For this review, take the finished solid that the model builds, in its own axes (mm). Face numbers are marked on the shaded views. A direction names the side the tool comes from. Coordinates: 2 decimals unless noted, no trailing zeros. Write each loop counter-clockwise with the first axis right and the second up, starting at its lowest first coordinate (ties: lowest second). Pieces come first, ordered by that corner, then holes.
1) We need section A-A on x = -0.5. Write out the cut boundary in (y, z).
2) We need section D-D on z = -57.5. Write out the cut boundary in (x, y), then the cut area to 3 significant figures.
3) To check wall thickness, follow line 1 along Y through (x, z) = (-0.5, 7); line 2 along Z through (x, y) = (-3.25, 13); line 3 along Y through (x, z) = (6.5, -11). State the ranges of each line that lie inside material, in increasing order.
4) For the marked faces 1, 2 and 3, list the 3-axis set-ups (+Z, -Z, +X, -X, +Y, -Y) from which the entire face can be reached by the end or side of a thin tool; tool diameter is ignored.
5) We need section B-B on z = -16. Write out the cut boundary in (x, y).
6) Insertion check: P1, Ø5, axis at x = -2.5, y = 17.5, coming from the -Z side; P2, Ø4, axis at x = 1, y = 26, coming from the -Z side; P3, Ø2, axis at x = 3.5, y = 24, coming from the +Z side. Each pin has a flat end and moves straight along its axis. Give the tip position at first contact, or say it passes through.
7) We need section C-C on y = 6. Write out the cut boundary in (x, z), then the cut area to 3 significant figures.
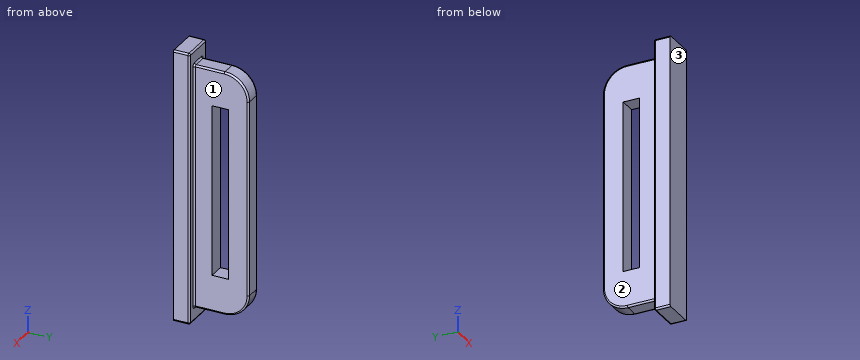
Autodesk Inventor part; units mm, degrees
ref_plane "YZ Plane" through (0, 0, 0) normal (1, 0, 0) x (0, 1, 0)
ref_plane "XZ Plane" through (0, 0, 0) normal (0, 1, 0) x (-1, 0, 0)
ref_plane "XY Plane" through (0, 0, 0) normal (0, 0, 1) x (1, 0, 0)
sketch "Sketch1" plane through (0, 0, 0) normal (1, 0, 0) x (0, 1, 0)
  line L0 (0, 76.2) -> (19.05, 76.2)
  line L1 (34.29, 60.96) -> (34.29, -60.96)
  line L2 (19.05, -76.2) -> (0, -76.2)
  line L3 (0, -76.2) -> (0, 76.2)
  line L4 (21.59, 53.34) -> (11.43, 53.34)
  line L5 (11.43, 53.34) -> (11.43, -53.34)
  line L6 (11.43, -53.34) -> (21.59, -53.34)
  line L7 (21.59, -53.34) -> (21.59, 53.34)
  line L8 (21.59, 53.34) -> (11.43, -53.34) construction
  line L9 (11.43, 53.34) -> (21.59, -53.34) construction
  arc A0 (34.29, 60.96) -> (19.05, 76.2) centre (19.05, 60.96) ccw
  arc A1 (19.05, -76.2) -> (34.29, -60.96) centre (19.05, -60.96) ccw
  line L10 (0, 0) -> (84.7989, 0) construction
  point P0 (16.51, 0)
  dimension "d0" = 15.24
  dimension "d1" = 152.4
  dimension "d2" = 106.68
  dimension "d3" = 34.29
  dimension "d4" = 11.43
  dimension "d5" = 10.16
extrude "Extrusion1" add sketch "Sketch1" along normal mid plane 10.16
sketch "Sketch3" plane through (0, 0, 0) normal (0, 1, 0) x (-1, 0, 0)
  line L0 (9.906, 85.09) -> (-9.906, 85.09)
  line L1 (-9.906, 85.09) -> (-9.906, -85.09)
  line L2 (-9.906, -85.09) -> (9.906, -85.09)
  line L3 (9.906, -85.09) -> (9.906, 85.09)
  line L4 (9.906, 85.09) -> (-9.906, -85.09) construction
  line L5 (-9.906, 85.09) -> (9.906, -85.09) construction
  point P0 (0, 0)
  dimension "d8" = 170.18
  dimension "d9" = 19.812
extrude "Extrusion2" add sketch "Sketch3" against normal blind 10.16
fillet "Fillet1" radius 1.016 22 edges at (5.08, 29.8263, 71.7363) (5.08, 9.525, 76.2) (5.08, 29.8263, -71.7363) (5.08, 9.525, -76.2) (5.08, 34.29, 0) (-5.08, 34.29, 0) (-5.08, 29.8263, -71.7363) (-5.08, 9.525, -76.2) (-5.08, 9.525, 76.2) (-5.08, 29.8263, 71.7363) (0, 0, 76.2) (5.08, 0, 0) (0, 0, -76.2) (-5.08, 0, 0) (0, 0, 85.09) (9.906, 0, 0) (-9.906, 0, 0) (9.906, -5.08, 85.09) (-9.906, -5.08, 85.09) (9.906, -5.08, -85.09) (0, 0, -85.09) (-9.906, -5.08, -85.09)
properties part number "Base"
Result:
1. outline: (-10.16, -85.09) - (-1.02, -85.09) arc R1.02 ccw to (0, -84.07) - (0, -77.22) arc R1.02 cw to (1.02, -76.2) - (19.05, -76.2) arc R15.24 ccw to (34.29, -60.96) - (34.29, 60.96) arc R15.24 ccw to (19.05, 76.2) - (1.02, 76.2) arc R1.02 cw to (0, 77.22) - (0, 84.07) arc R1.02 ccw to (-1.02, 85.09) - (-10.16, 85.09) - close; hole (11.43, -53.34) - (21.59, -53.34) - (21.59, 53.34) - (11.43, 53.34) - close
2. outline: (-9.91, -10.16) - (9.91, -10.16) - (9.91, -1.02) arc R1.02 ccw to (8.89, 0) - (6.1, 0) arc R1.02 cw to (5.08, 1.02) - (5.08, 33.27) arc R1.02 ccw to (4.06, 34.29) - (-4.06, 34.29) arc R1.02 ccw to (-5.08, 33.27) - (-5.08, 1.02) arc R1.02 cw to (-6.1, 0) - (-8.89, 0) arc R1.02 ccw to (-9.91, -1.02) - close
2. area: 549 mm2
3. line 1: y = -10.16 to 11.43, 21.59 to 34.29
3. line 2: z = -76.2 to -53.34, 53.34 to 76.2
3. line 3: y = -10.16 to 0
4. face 1: +Z, -Z, +X, +Y
4. face 2: +Z, -Z, -X, +Y
4. face 3: +Z, -Z, +X, -X, -Y
5. outline: (-9.91, -10.16) - (9.91, -10.16) - (9.91, -1.02) arc R1.02 ccw to (8.89, 0) - (6.1, 0) arc R1.02 cw to (5.08, 1.02) - (5.08, 11.43) - (-5.08, 11.43) - (-5.08, 1.02) arc R1.02 cw to (-6.1, 0) - (-8.89, 0) arc R1.02 ccw to (-9.91, -1.02) - close; (-5.08, 21.59) - (5.08, 21.59) - (5.08, 33.27) arc R1.02 ccw to (4.06, 34.29) - (-4.06, 34.29) arc R1.02 ccw to (-5.08, 33.27) - close
6. P1: stops at z = -76.2
6. P2: stops at z = -75.37
6. P3: stops at z = 75.68
7. outline: (-5.08, -75.18) arc R1.02 ccw to (-4.06, -76.2) - (4.06, -76.2) arc R1.02 ccw to (5.08, -75.18) - (5.08, 75.18) arc R1.02 ccw to (4.06, 76.2) - (-4.06, 76.2) arc R1.02 ccw to (-5.08, 75.18) - close
7. area: 1,550 mm2
